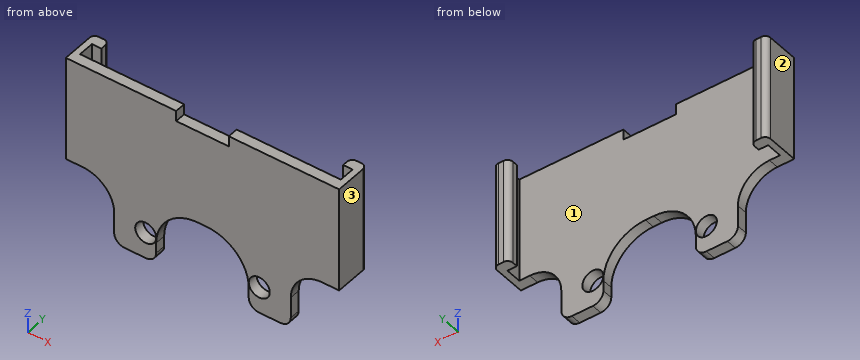
```python
from build123d import *

# Parameters (mm, degrees)
EXTRUDE_1_DEPTH     = 1
SKETCH_3_R          = 1
CUT_EXTRUDE_3_DEPTH = 21.639767441
SKETCH_6_W          = 5
SKETCH_6_H          = 2
CUT_EXTRUDE_4_DEPTH = 21.639767441
SKETCH_7_W          = 0.6
SKETCH_7_H          = 10
EXTRUDE_2_DEPTH     = 1.5
SKETCH_8_W          = 1.5
SKETCH_8_H          = 10
EXTRUDE_3_DEPTH     = 1
FILLET_1_R          = 0.5


with BuildPart() as part:
    # Эскиз1 → Бобышка-Вытянуть1 (new body)
    with BuildSketch(Plane(origin=(0, 0, 0), x_dir=(1, 0, 0), z_dir=(0, 1, 0))):
        with BuildLine():
            Line((-7.4, 16), (-5.4, 16))
            ThreePointArc((-5.4, 16), (-4.692893219, 15.707106781), (-4.4, 15))
            Line((-4.4, 15), (-4.4, 14))
            ThreePointArc((-4.4, 14), (-3.228427125, 11.171572875), (-0.4, 10))
            Line((-0.4, 10), (0.4, 10))
            ThreePointArc((0.4, 10), (3.228427125, 11.171572875), (4.4, 14))
            Line((4.4, 14), (4.4, 15))
            ThreePointArc((4.4, 15), (4.692893219, 15.707106781), (5.4, 16))
            Line((5.4, 16), (7.4, 16))
            ThreePointArc((7.4, 16), (8.107106781, 15.707106781), (8.4, 15))
            Line((8.4, 15), (8.4, 13))
            ThreePointArc((8.4, 13), (9.278679656, 10.878679656), (11.4, 10))
            Line((11.4, 10), (13, 10))
            Line((13, 10), (13, 0))
            Line((13, 0), (-13, 0))
            Line((-13, 0), (-13, 10))
            Line((-13, 10), (-11.4, 10))
            ThreePointArc((-11.4, 10), (-9.278679656, 10.878679656), (-8.4, 13))
            Line((-8.4, 13), (-8.4, 15))
            ThreePointArc((-8.4, 15), (-8.107106781, 15.707106781), (-7.4, 16))
        make_face()
    extrude(amount=-EXTRUDE_1_DEPTH)

    # Эскиз3 → Вырез-Вытянуть3 (cut, through all)
    with BuildSketch(Plane(origin=(0, 0, 0), x_dir=(1, 0, 0), z_dir=(0, 1, 0))):
        with Locations(Location((-5.4, 13.5, 0), (0, 0, 270))):
            Circle(SKETCH_3_R)
        with Locations(Location((5.4, 13.5, 0), (0, 0, 270))):
            Circle(SKETCH_3_R)
    extrude(amount=-CUT_EXTRUDE_3_DEPTH, mode=Mode.SUBTRACT)

    # Эскиз6 → Вырез-Вытянуть4 (cut, through all)
    with BuildSketch(Plane(origin=(0, 0, 0), x_dir=(1, 0, 0), z_dir=(0, 1, 0))):
        Rectangle(SKETCH_6_W, SKETCH_6_H)
    extrude(amount=-CUT_EXTRUDE_4_DEPTH, mode=Mode.SUBTRACT)

    # Эскиз7 → Бобышка-Вытянуть2 (add)
    with BuildSketch(Plane(origin=(0, 0, 0), x_dir=(1, 0, 0), z_dir=(0, 1, 0))):
        with Locations((-12.7, 5)):
            Rectangle(SKETCH_7_W, SKETCH_7_H)
        with Locations((12.7, 5)):
            Rectangle(SKETCH_7_W, SKETCH_7_H)
    extrude(amount=EXTRUDE_2_DEPTH)

    # Эскиз8 → Бобышка-Вытянуть3 (add)
    with BuildSketch(Plane(origin=(0, 1.5, 0), x_dir=(1, 0, 0), z_dir=(0, 1, 0))):
        with Locations((-12.25, 5)):
            Rectangle(SKETCH_8_W, SKETCH_8_H)
        with Locations((12.25, 5)):
            Rectangle(SKETCH_8_W, SKETCH_8_H)
    extrude(amount=EXTRUDE_3_DEPTH)

    # Скругление1
    fillet_1_edges = [part.edges().sort_by_distance(p)[0] for p in [
        (-13, 2.5, -5),
        (-11.5, 2.5, -5),
        (13, 2.5, -5),
        (11.5, 2.5, -5),
    ]]
    fillet(fillet_1_edges, radius=FILLET_1_R)


solid = part.part
```
Model file for the job. Use its own axes, mm. Face numbers are marked on the shaded views. Coordinates: 2 decimals unless noted, no trailing zeros. Write each loop counter-clockwise with the first axis right and the second up, starting at its lowest first coordinate (ties: lowest second). Pieces come first, ordered by that corner, then holes. Notation, with made-up numbers: (14, 11.25) - (45, 11.25) arc R5 cw to (45, 16.25) - close; hole circle Ø1 at (89.5, 43.5). An arc over 180 degrees is marked (long way). One line per item, written item: value. Start each with the question number.
1. Slice it at A-A (y = 0.8). Write the cut outline in (x, z).
2. Flat gauge pins, fed straight in: pin 1 (0.5 mm diameter, centred on y = -0.5, z = -14, fed in from +X); pin 2 (0.8 mm diameter, centred on x = 12, y = 1.5, fed in from -Z); pin 3 (5 mm diameter, centred on x = -4, z = -11, fed in from +Y). Where does each tip first touch, or does it go through?
3. Probe line 1 (X direction, y = 1.55, z = -2.75); line 2 (X direction, y = -0.6, z = -0.75); line 3 (Y direction, x = 6.75, z = -12.5). List the from-to ranges inside material, lowest first. Write a range as from..to.
4. Slice it at C-C (z = -3.75). Write the cut outline in (x, y).
5. Slice it at B-B (z = -13.75). Count the separate pieces of the cut face and the enclosed holes in it, plus the area to 3 significant figures.
6. Mould opens along X. For the marked faces 1, 2 and 3 say: released by +X, released by -X, zero draft, split by the parting line, or undercut.
7. Slice it at D-D (x = -3). Write the cut outline in (y, z).
Answers below:
1. outline: (-13, -10) - (-12.4, -10) - (-12.4, 0) - (-13, 0) - close; (12.4, -10) - (13, -10) - (13, 0) - (12.4, 0) - close
2. pin 1: stops at x = 8.4
2. pin 2: stops at z = -10
2. pin 3: stops at y = 0
3. line 1: x = -13..-11.5, 11.5..13
3. line 2: x = -13..-2.5, 2.5..13
3. line 3: y = -1..0
4. outline: (-13, -1) - (13, -1) - (13, 2) arc R0.5 ccw to (12.5, 2.5) - (12, 2.5) arc R0.5 ccw to (11.5, 2) - (11.5, 1.5) - (12.4, 1.5) - (12.4, 0) - (-12.4, 0) - (-12.4, 1.5) - (-11.5, 1.5) - (-11.5, 2) arc R0.5 ccw to (-12, 2.5) - (-12.5, 2.5) arc R0.5 ccw to (-13, 2) - close
5. separate pieces: 4
5. enclosed holes: 0
5. area: 4.14 mm^2
6. face 1: undercut
6. face 2: released by -X
6. face 3: released by +X
7. outline: (-1, -10.96) - (0, -10.96) - (0, 0) - (-1, 0) - close
